from build123d import *

# Parameters (mm, degrees)
SKETCH1_R           = 85.725
BOSS_EXTRUDE1_DEPTH = 12.7
BOSS_EXTRUDE2_DEPTH = 6.35
SKETCH3_R           = 6.35
SKETCH3_R_2         = 5.08
BOSS_EXTRUDE3_DEPTH = 6.096
SKETCH4_W           = 21.0058
SKETCH4_H           = 34.925
CUT_EXTRUDE1_DEPTH  = 9.525


with BuildPart() as part:
    # Sketch1 → Boss-Extrude1 (new body)
    with BuildSketch(Plane(origin=(0, 0, 0), x_dir=(1, 0, 0), z_dir=(0, 1, 0))):
        Circle(SKETCH1_R)
    extrude(amount=BOSS_EXTRUDE1_DEPTH)

    # Sketch2 → Boss-Extrude2 (add)
    with BuildSketch(Plane(origin=(0, 12.7, 0), x_dir=(1, 0, 0), z_dir=(0, 1, 0))):
        Polygon((-25.4, 81.875610685), (25.4, 81.875610685), (85.725, 0), (0, -85.725), (-85.725, 0), align=None)
    extrude(amount=BOSS_EXTRUDE2_DEPTH)

    # Sketch3 → Boss-Extrude3 (add)
    with BuildSketch(Plane(origin=(0, 12.7, 0), x_dir=(1, 0, 0), z_dir=(0, 1, 0))):
        with Locations((-51.739614409, -51.739614409)):
            Circle(SKETCH3_R)
        with Locations((51.739614409, -51.739614409)):
            Circle(SKETCH3_R)
        with Locations((62.288840877, 45.893695259)):
            Circle(SKETCH3_R_2)
        with Locations((-62.288840877, 45.893695259)):
            Circle(SKETCH3_R_2)
    extrude(amount=BOSS_EXTRUDE3_DEPTH)

    # Sketch4 → Cut-Extrude1 (cut)
    with BuildSketch(Plane(origin=(0, 19.05, 0), x_dir=(1, 0, 0), z_dir=(0, 1, 0))):
        with Locations((0, 51.713110685)):
            Rectangle(SKETCH4_W, SKETCH4_H)
    extrude(amount=-CUT_EXTRUDE1_DEPTH, mode=Mode.SUBTRACT)


solid = part.part
Can you work these out from the model? Positions are in its coordinate system, mm. A direction names the side the tool comes from. Give positions to 0.01 mm unless a question says otherwise; leave off trailing zeros. Loops run counter-clockwise (first coordinate to the right, second up) from the corner with the lowest first, then second, coordinate; pieces in that order, holes last. Notation, with made-up numbers: M 88.25,-18 L 132.25,-18 A15 cw 132.25,-5 Z; hole C 30.5,14 d7. An arc over 180 degrees is marked long. One line per item, written item: value. Start each with the question number.
1) I'm going to push flat-ended pins straight in: pin 1 (10 mm diameter, centred on x = -50, z = 53.5, fed in from +Y); pin 2 (5 mm diameter, centred on x = -6.5, y = 16, fed in from -Z); pin 3 (10 mm diameter, centred on y = 14, z = -13, fed in from +X). Where does each tip first touch, or does it pass through?
2) If I drill on line 1 (Y direction, x = 61, z = 42); line 2 (Z direction, x = -7, y = 17.5) (3 decimals); line 3 (X direction, y = 16, z = -53), over which ranges is the centre line in solid material (lowest first)? Write a range as [from, to].
3) Thinking about a two-plate mould opening in X: for faces 4 (the face through (46.09, 6.26, -72.28)), 5 (the face through (-62.95, 15.71, -50.93)), 6 (the face through (55.14, 15.83, -41.51)), 7 (the face through (-62, 18.796, -46)), which applies, +X half, -X half, draft (parallel to the pull), parting line (faces both ways), or undercut?
4) If we section it at D-D, the plane z = -66: Write out the boundary of the cut face in (x, y) (3 decimals), and give its area (3 significant figures).
5) If we section it at B-B, the plane x = 41: Write out the boundary of the cut face in (y, z) (3 decimals), and give its area (3 significant figures).
6) On a 3-axis mill with a long thin cutter (end or side, diameter ignored), from which of +Z, -Z, +X, -X, +Y, -Y can I reach the whole of each face in a straight line? I mean faces 1 (the face through (0, 12.7, -83)), 2 (the face through (62, 18.796, -46)), 3 (the face through (-52, 18.796, 52)). Say none if no direction works.
7) If we section it at C-C, the plane y = 4: Write out the boundary of the cut face in (x, z) (3 decimals), and give its area (3 significant figures).
8) If we section it at A-A, the plane z = 75.5: Write out the boundary of the cut face in (x, y) (3 decimals).
Completed:
1. pin 1: stops at y = 18.8
1. pin 2: stops at z = -81.88
1. pin 3: stops at x = 85.33
2. line 1: y = [0, 12.7]
2. line 2: z = [-81.876, -69.176], [-34.251, 78.725]
2. line 3: x = [-46.68, -10.5], [10.5, 46.68]
3. face 4: parting line
3. face 5: undercut
3. face 6: undercut
3. face 7: draft
4. outline: M -54.706,0 L 54.706,0 L 54.706,12.7 L 37.097,12.7 L 37.097,19.05 L 10.503,19.05 L 10.503,9.525 L -10.503,9.525 L -10.503,19.05 L -37.097,19.05 L -37.097,12.7 L -54.706,12.7 Z
4. area: 1,660 mm^2
5. outline: M 0,-75.285 L 12.7,-75.285 L 12.7,-60.703 L 19.05,-60.703 L 19.05,44.725 L 12.7,44.725 L 12.7,75.285 L 0,75.285 Z
5. area: 2,580 mm^2
6. face 1: -Z, +X, -X, +Y
6. face 2: -Z, +X, +Y
6. face 3: +Z, -X, +Y
7. outline: C 0,0 d171.45
7. area: 23,100 mm^2
8. outline: M -40.602,0 L 40.602,0 L 40.602,12.7 L 10.225,12.7 L 10.225,19.05 L -10.225,19.05 L -10.225,12.7 L -40.602,12.7 Z
